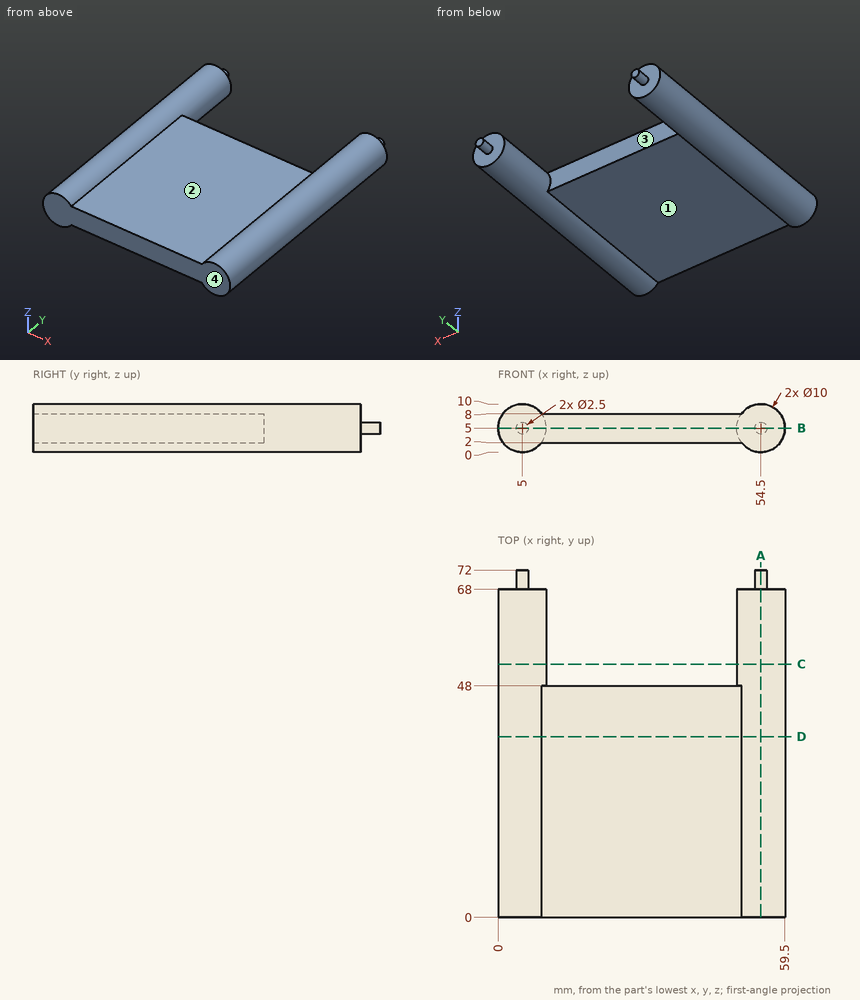
Study the drawing (mm; zero at the part's minimum x, y, z) and answer. A direction names the side the tool comes from. Coordinates: 2 decimals unless noted, no trailing zeros. Write each loop counter-clockwise with the first axis right and the second up, starting at its lowest first coordinate (ties: lowest second). Pieces come first, ordered by that corner, then holes. Notation, with made-up numbers: M 65.5,77.5 L 119.5,77.5 A27 cw 119.5,97.5 Z; hole C 13.25,75 d9. An arc over 180 degrees is marked long. Use a Markdown table: item, result. Add a question column.
1. Section A-A (x = 54.5) is taken. Give the vertices of the cut face in (y, z).
2. Straight lines are drawn through the part: line 1 along Z through (x, y) = (25.5, 5.5); line 2 along Y through (x, z) = (45, 6.5); line 3 along Y through (x, z) = (9.5, 3). For each, find the intervals that lie inside material, in ascending order. Write a range as [from, to].
3. Which of the six approach directions +Z, -Z, +X, -X, +Y, -Y give full straight-line access (tool end or side, diameter ignored) to the marked faces 1 and 2?
4. Given P1, Ø1, axis at y = 41.5, z = 4, coming from the +X side; P2, Ø20.5, axis at x = 19.5, y = 15, coming from the -Z side; P3, Ø5, axis at x = 8.5, y = 38, coming from the +Z side, each flat-ended and moving along its own axis, determine where each tip first touches the part or whether it passes through.
5. Section C-C (y = 52.5) is taken. Give the vertices of the cut face in (x, z), plus the area to 3 significant figures.
6. Section B-B (z = 5) is taken. Give the vertices of the cut face in (x, y).
7. Section D-D (y = 37.5) is taken. Give the vertices of the cut face in (x, z).
8. For a pull along X with two mould halves and no side action, classify the marked faces 3 and 4 as +X half, -X half, draft (parallel to the pull), parting line (faces both ways), or undercut.
Data:
| question | item | result |
|---|---|---|
| 1 | outline | M 0,0 L 68,0 L 68,3.75 L 72,3.75 L 72,6.25 L 68,6.25 L 68,10 L 0,10 Z |
| 2 | line 1 | z = [2, 8] |
| 2 | line 2 | y = [0, 48] |
| 2 | line 3 | y = [0, 68] |
| 3 | face 1 | -Z, +Y, -Y |
| 3 | face 2 | +Z, +Y, -Y |
| 4 | P1 | stops at x = 59.47 |
| 4 | P2 | stops at z = 2 |
| 4 | P3 | stops at z = 9.9 |
| 5 | outline | C 5,5 d10; C 54.5,5 d10 |
| 5 | area | 157 mm2 |
| 6 | outline | M 0,0 L 59.5,0 L 59.5,68 L 55.75,68 L 55.75,72 L 53.25,72 L 53.25,68 L 49.5,68 L 49.5,48 L 10,48 L 10,68 L 6.25,68 L 6.25,72 L 3.75,72 L 3.75,68 L 0,68 Z |
| 7 | outline | M 9,2 L 50.5,2 A5 ccw long 50.5,8 L 9,8 A5 ccw long Z |
| 8 | face 3 | undercut |
| 8 | face 4 | draft |
